Design review of the part built by this model. Coordinates are the model's own, in mm. Give positions to 0.01 mm unless a question says otherwise; leave off trailing zeros. Order: outer loops, then holes, each group sorted by start corner. A loop starts at its lowest first (then second) coordinate and runs counter-clockwise, first axis right, second up. Notation, with made-up numbers: M 74,80.5 L 133,80.5 A12 cw 133,102.5 Z; hole C 74.5,-1 d6. An arc over 180 degrees is marked long. Answer as a JSON object with one key per item and string values.
from build123d import *

# Parameters (mm, degrees)
SKETCH1_R           = 3.25
SKETCH1_R_2         = 1.5
BOSS_EXTRUDE1_DEPTH = 3


with BuildPart() as part:
    # Sketch1 → Boss-Extrude1 (new body)
    with BuildSketch(Plane(origin=(0, 0, 0), x_dir=(-1, 0, 0), z_dir=(0, 0, -1))):
        with BuildLine():
            Line((8.181538342, 15.560412846), (11.282357346, 86.580844321))
            ThreePointArc((11.282357346, 86.580844321), (11.19104264, 87.774392868), (10.818655174, 88.912032567))
            Line((10.818655174, 88.912032567), (7.70361619, 95.592255225))
            ThreePointArc((7.70361619, 95.592255225), (0, 100.5), (-7.70361619, 95.592255225))
            Line((-7.70361619, 95.592255225), (-10.818655174, 88.912032567))
            ThreePointArc((-10.818655174, 88.912032567), (-11.19104264, 87.774392868), (-11.282357346, 86.580844321))
            Line((-11.282357346, 86.580844321), (-8.181538342, 15.560412846))
            ThreePointArc((-8.181538342, 15.560412846), (-8.600305132, 13.328393664), (-9.963157432, 11.511828536))
            ThreePointArc((-9.963157432, 11.511828536), (-12.324154236, 8.321537367), (-12.979294427, 4.407069973))
            Line((-12.979294427, 4.407069973), (-12.122281745, -7.848782369))
            ThreePointArc((-12.122281745, -7.848782369), (-11.79450084, -9.312190191), (-11.047502278, -10.612573183))
            Line((-11.047502278, -10.612573183), (-8.26347657, -14.112573183))
            ThreePointArc((-8.26347657, -14.112573183), (-6.522662073, -15.503491197), (-4.350435786, -16))
            Line((-4.350435786, -16), (4.350435786, -16))
            ThreePointArc((4.350435786, -16), (6.522662073, -15.503491197), (8.26347657, -14.112573183))
            Line((8.26347657, -14.112573183), (11.047502278, -10.612573183))
            ThreePointArc((11.047502278, -10.612573183), (11.79450084, -9.312190191), (12.122281745, -7.848782369))
            Line((12.122281745, -7.848782369), (12.979294427, 4.407069973))
            ThreePointArc((12.979294427, 4.407069973), (12.324154236, 8.321537367), (9.963157432, 11.511828536))
            ThreePointArc((9.963157432, 11.511828536), (8.600305132, 13.328393664), (8.181538342, 15.560412846))
        make_face()
        with Locations(Location((0, 0, 0), (0, 0, 180))):
            Circle(SKETCH1_R, mode=Mode.SUBTRACT)
        with Locations(Location((6.25, 89, 0), (0, 0, 180))):
            Circle(SKETCH1_R_2, mode=Mode.SUBTRACT)
        with Locations(Location((6.25, 79, 0), (0, 0, 180))):
            Circle(SKETCH1_R_2, mode=Mode.SUBTRACT)
        with Locations(Location((-6.25, 89, 0), (0, 0, 180))):
            Circle(SKETCH1_R_2, mode=Mode.SUBTRACT)
        with Locations(Location((-6.25, 79, 0), (0, 0, 180))):
            Circle(SKETCH1_R_2, mode=Mode.SUBTRACT)
        with BuildLine():
            Line((7.778174593, 6.01040764), (5.656854249, 3.889087297))
            ThreePointArc((5.656854249, 3.889087297), (3.889087297, 3.889087297), (3.889087297, 5.656854249))
            Line((3.889087297, 5.656854249), (6.01040764, 7.778174593))
            ThreePointArc((6.01040764, 7.778174593), (7.778174593, 7.778174593), (7.778174593, 6.01040764))
        make_face(mode=Mode.SUBTRACT)
        with BuildLine():
            Line((-5.656854249, 3.889087297), (-7.778174593, 6.01040764))
            ThreePointArc((-7.778174593, 6.01040764), (-7.778174593, 7.778174593), (-6.01040764, 7.778174593))
            Line((-6.01040764, 7.778174593), (-3.889087297, 5.656854249))
            ThreePointArc((-3.889087297, 5.656854249), (-3.889087297, 3.889087297), (-5.656854249, 3.889087297))
        make_face(mode=Mode.SUBTRACT)
        with BuildLine():
            Line((-3.889087297, -5.656854249), (-6.01040764, -7.778174593))
            ThreePointArc((-6.01040764, -7.778174593), (-7.778174593, -7.778174593), (-7.778174593, -6.01040764))
            Line((-7.778174593, -6.01040764), (-5.656854249, -3.889087297))
            ThreePointArc((-5.656854249, -3.889087297), (-3.889087297, -3.889087297), (-3.889087297, -5.656854249))
        make_face(mode=Mode.SUBTRACT)
        with BuildLine():
            Line((6.01040764, -7.778174593), (3.889087297, -5.656854249))
            ThreePointArc((3.889087297, -5.656854249), (3.889087297, -3.889087297), (5.656854249, -3.889087297))
            Line((5.656854249, -3.889087297), (7.778174593, -6.01040764))
            ThreePointArc((7.778174593, -6.01040764), (7.778174593, -7.778174593), (6.01040764, -7.778174593))
        make_face(mode=Mode.SUBTRACT)
    extrude(amount=-BOSS_EXTRUDE1_DEPTH)


solid = part.part
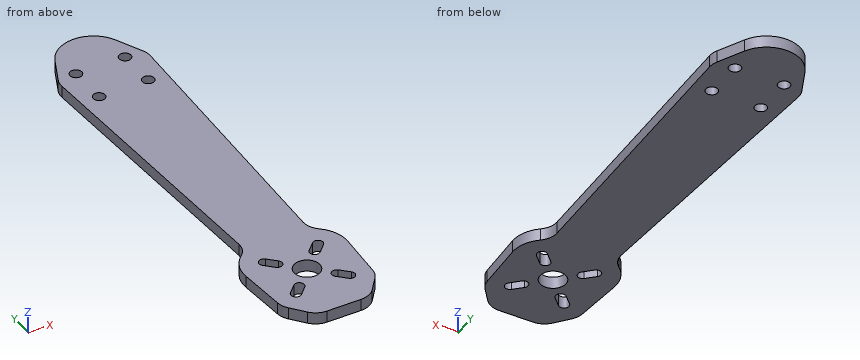
(1) To check wall thickness, follow L1, parallel to X at y = 89, z = 1.05; L2, parallel to Y at x = -6.25, z = 1.95; L3, parallel to X at y = 79, z = 1.7. State the ranges of each line that lie inside material, in increasing order. Write a range as from..to.
Checked values:
{"L1": "x = -10.78..-7.75, -4.75..4.75, 7.75..10.78", "L2": "y = -15.63..-7.97, -4.48..4.48, 7.97..77.5, 80.5..87.5, 90.5..97.76", "L3": "x = -10.95..-7.75, -4.75..4.75, 7.75..10.95"}
(2) We need section A-A (x = 0). Write out the cut boundary in (y, z), plus the area to 3 significant figures.
Checked values:
{"outline": "M -16,0 L -3.25,0 L -3.25,3 L -16,3 Z; M 3.25,0 L 100.5,0 L 100.5,3 L 3.25,3 Z", "area": "330 mm^2"}
(3) We need section C-C (y = 79). Write out the cut boundary in (x, z).
Checked values:
{"outline": "M -10.95,0 L -7.75,0 L -7.75,3 L -10.95,3 Z; M -4.75,0 L 4.75,0 L 4.75,3 L -4.75,3 Z; M 7.75,0 L 10.95,0 L 10.95,3 L 7.75,3 Z"}
(4) We need section D-D (z = 0.65). Count the separate pieces of the cut face and the enclosed holes in it, plus the area to 3 significant figures.
Checked values:
{"separate pieces": "1", "enclosed holes": "9", "area": "2,210 mm^2"}
(5) We need section B-B (y = 0). Write out the cut boundary in (x, z).
Checked values:
{"outline": "M -12.67,0 L -3.25,0 L -3.25,3 L -12.67,3 Z; M 3.25,0 L 12.67,0 L 12.67,3 L 3.25,3 Z"}
